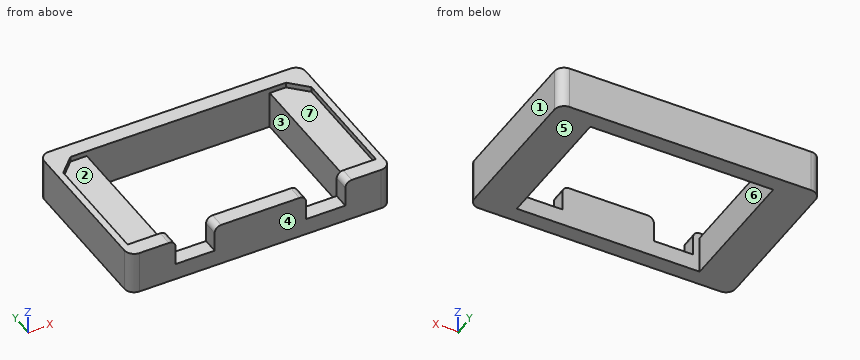
```python
from build123d import *

# Parameters (mm, degrees)
F0_W     = 80
F0_H     = 50
F1_DEPTH = 11.5
F2_W     = 80
F2_H     = 50
F3_DEPTH = 1.6
F4_W     = 56
F4_H     = 40.5
F5_DEPTH = 11.5
F6_W     = 12
F6_H     = 4.75
F7_DEPTH = 8
F8_R     = 3
F9_R     = 2


with BuildPart() as f1:
    # F0 (on Top) → F1 (new body)
    with BuildSketch(Plane.XY):
        Rectangle(F0_W, F0_H)
    extrude(amount=-F1_DEPTH)

    # F2 (on face) → F3 (join)
    with BuildSketch(Plane.XY):
        Rectangle(F2_W, F2_H)
        Polygon((38, -20.25), (-38, -20.25), (-38, 15.25), (-33, 20.25), (33, 20.25), (38, 15.25), align=None, mode=Mode.SUBTRACT)
    extrude(amount=F3_DEPTH)

    # F4 (on face) → F5 (cut, through all)
    with BuildSketch(Plane.XY):
        Rectangle(F4_W, F4_H)
    extrude(amount=-F5_DEPTH, mode=Mode.SUBTRACT)

    # F6 (on face) → F7 (cut)
    with BuildSketch(Plane.XY.offset(1.6)):
        with Locations((-20, -22.625)):
            Rectangle(F6_W, F6_H)
        with Locations((20, -22.625)):
            Rectangle(F6_W, F6_H)
    extrude(amount=-F7_DEPTH, mode=Mode.SUBTRACT)

    # F8
    f8_edges = [f1.edges().sort_by_distance(p)[0] for p in [
        (-40, 25, -4.95),
        (-40, -25, -4.95),
        (40, -25, -4.95),
        (40, 25, -4.95),
    ]]
    fillet(f8_edges, radius=F8_R)

    # F9
    f9_edges = [f1.edges().sort_by_distance(p)[0] for p in [
        (-26, -22.625, 1.6),
        (-14, -22.625, 1.6),
        (14, -22.625, 1.6),
        (26, -22.625, 1.6),
    ]]
    fillet(f9_edges, radius=F9_R)


solid = f1.part
```
Part model, mm, in its own coordinate system. Face numbers are marked on the shaded views. A direction names the side the tool comes from. Round coordinates to 2 decimals unless told otherwise and drop trailing zeros. Loops run counter-clockwise (first coordinate to the right, second up) from the corner with the lowest first, then second, coordinate; pieces in that order, holes last. Notation, with made-up numbers: (47.25, 22) -> (84.25, 22) arc R22 cw to (84.25, 44) -> close; hole circle Ø8 at (73.25, 61.5). An arc over 180 degrees is marked (long way). Use a Markdown table: item, result.
1) Cut at B-B, the plane y = 19. List the corners of the cut face in (x, z).
The answers:
| item | result |
|---|---|
| outline | (-40, -11.5) -> (-28, -11.5) -> (-28, 0) -> (-34.25, 0) -> (-34.25, 1.6) -> (-40, 1.6) -> close; (28, -11.5) -> (40, -11.5) -> (40, 1.6) -> (34.25, 1.6) -> (34.25, 0) -> (28, 0) -> close |
2) Probe line 1 (Y direction, x = -25.5, z = -9.5); line 2 (X direction, y = 0, z = -10.5); line 3 (Y direction, x = -34, z = 0.5). List the from-to ranges inside material, lowest first. Write a range as [from, to].
The answers:
| item | result |
|---|---|
| line 1 | y = [-25, -20.25], [20.25, 25] |
| line 2 | x = [-40, -28], [28, 40] |
| line 3 | y = [-25, -20.25], [19.25, 25] |
3) Cut at A-A, the plane z = -2. List the corners of the cut face in (x, y).
The answers:
| item | result |
|---|---|
| outline | (-40, -22) arc R3 ccw to (-37, -25) -> (-26, -25) -> (-26, -20.25) -> (-28, -20.25) -> (-28, 20.25) -> (28, 20.25) -> (28, -20.25) -> (26, -20.25) -> (26, -25) -> (37, -25) arc R3 ccw to (40, -22) -> (40, 22) arc R3 ccw to (37, 25) -> (-37, 25) arc R3 ccw to (-40, 22) -> close; (-14, -25) -> (14, -25) -> (14, -20.25) -> (-14, -20.25) -> close |
4) Pull direction Y, two halves, no side cores. Call the marked faces 1, 2, 3 and 4: pulls with the +Y half, pulls with the -Y half, needs draft (parallel to the pull), parting line crosses it, or undercut.
The answers:
| item | result |
|---|---|
| face 1 | needs draft |
| face 2 | undercut |
| face 3 | undercut |
| face 4 | pulls with the -Y half |
5) Tool access for the marked faces 5, 6 and 7: list every direction of +Z, -Z, +X, -X, +Y, -Y with a clear straight run to the whole face (end or side of a thin tool).
The answers:
| item | result |
|---|---|
| face 5 | -Z, +X, -X, +Y, -Y |
| face 6 | +Z, -Z |
| face 7 | +Z |
6) Cut at D-D, the plane z = -9.75. List the corners of the cut face in (x, y), and give its area (3 significant figures).
The answers:
| item | result |
|---|---|
| outline | (-40, -22) arc R3 ccw to (-37, -25) -> (37, -25) arc R3 ccw to (40, -22) -> (40, 22) arc R3 ccw to (37, 25) -> (-37, 25) arc R3 ccw to (-40, 22) -> close; hole (-28, -20.25) -> (28, -20.25) -> (28, 20.25) -> (-28, 20.25) -> close |
| area | 1,720 mm2 |
7) Cut at C-C, the plane x = 21. List the corners of the cut face in (y, z).
The answers:
| item | result |
|---|---|
| outline | (-25, -11.5) -> (-20.25, -11.5) -> (-20.25, -6.4) -> (-25, -6.4) -> close; (20.25, -11.5) -> (25, -11.5) -> (25, 1.6) -> (20.25, 1.6) -> close |
8) Drop flat-ended pins along their axis: pin 1 Ø5 at (x, y) = (31.5, 10) entering from +Z; pin 2 Ø1.4 at (x, y) = (21, -23) entering from +Z; pin 3 Ø2.5 at (y, z) = (-23.5, -3) entering from +X. Give the stop position or say it passes through.
The answers:
| item | result |
|---|---|
| pin 1 | stops at z = 0 |
| pin 2 | stops at z = -6.4 |
| pin 3 | stops at x = 39.99 |
